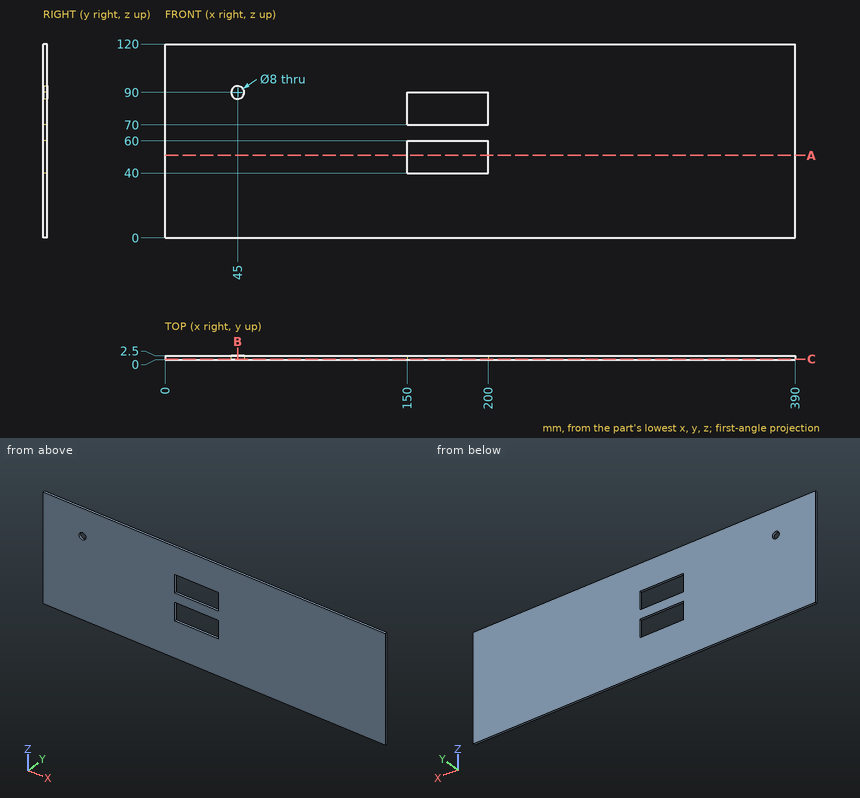
Can you work these out from the drawing? Everything is in mm from the part's minimum corner. Round coordinates to 2 decimals unless told otherwise and drop trailing zeros. Loops run counter-clockwise (first coordinate to the right, second up) from the corner with the lowest first, then second, coordinate; pieces in that order, holes last. Notation, with made-up numbers: (13.5, 23) - (69.5, 23) arc R16 ccw to (69.5, 39) - close; hole circle Ø11 at (60.25, -25). An arc over 180 degrees is marked (long way). One line per question, with ' | ' between items. Start each with the question number.
Q1. I want a section at A-A (z = 51). Write out the boundary of the cut face in (x, y).
Q2. Please list where these lines run through material, in increasing order: line 1 (Z direction, x = 152, y = 2.3); line 2 (X direction, y = 1.8, z = 54.5); line 3 (Z direction, x = 45, y = 1.8). Write a range as [from, to].
Q3. I want a section at B-B (x = 45). Write out the boundary of the cut face in (y, z).
Q4. I want a section at C-C (y = 0.45). Write out the boundary of the cut face in (x, z).
Response values:
1) outline: (0, 0) - (150, 0) - (150, 2.5) - (0, 2.5) - close; (200, 0) - (390, 0) - (390, 2.5) - (200, 2.5) - close
2) line 1: z = [0, 40], [60, 70], [90, 120] | line 2: x = [0, 150], [200, 390] | line 3: z = [0, 86], [94, 120]
3) outline: (0, 0) - (2.5, 0) - (2.5, 86) - (0, 86) - close; (0, 94) - (2.5, 94) - (2.5, 120) - (0, 120) - close
4) outline: (0, 0) - (390, 0) - (390, 120) - (0, 120) - close; hole circle Ø8 at (45, 90); hole (150, 40) - (200, 40) - (200, 60) - (150, 60) - close; hole (150, 70) - (200, 70) - (200, 90) - (150, 90) - close
